For this review, take the finished solid that the model builds, in its own axes (mm). A direction names the side the tool comes from. Coordinates: 2 decimals unless noted, no trailing zeros. Write each loop counter-clockwise with the first axis right and the second up, starting at its lowest first coordinate (ties: lowest second). Pieces come first, ordered by that corner, then holes. Notation, with made-up numbers: (-32, 76.25) -> (2, 76.25) arc R18 ccw to (2, 93.25) -> close; hole circle Ø4 at (-1, -20). An arc over 180 degrees is marked (long way). One line per item, written item: value. Start each with the question number.
1) Add section A-A (x = 300.75). State how many separate pieces and enclosed holes the cut face has, and give its area (3 significant figures).
2) Add section D-D (x = 36). State the section outline as (y, z) points.
3) Mouldability with a two-part tool opening along Y and no side actions: class faces 6 (the flat face through (149, 220, 20)), 7 (the flat face through (115, 0.25, 2)), 8 (the flat face through (209, -4, 40)) as released by +Y, released by -Y, zero draft, split by the parting line, or undercut.
4) For pin 1 Ø6 at (x, z) = (243, 10.5) entering from -Y; pin 2 Ø5 at (x, z) = (136.66, 36.28) entering from +Y; pin 3 Ø6 at (x, y) = (144, 62) entering from +Z; pin 4 Ø10 at (x, z) = (360, 27.5) entering from +Y, all flat-tipped, find the tip position at first contact; note any pin that passes through.
5) Machinability: for faces 1 (the flat face through (424.5, 108, 20)), 2 (the flat face through (213, -5, 41)), 3 (the flat face through (215, 225, 1)), 4 (the flat face through (420, -4, 0.75)), 5 (the flat face through (424.75, 109, 20)), which of the approach directions +Z, -Z, +X, -X, +Y, -Y give a long, thin tool a straight path to every point of the face, cutting with its end or side? Answer none if there is none.
6) For probe 1 along Y at (x, z) = (92, 36); probe 2 along X at (y, z) = (16.5, 38.5); probe 3 along Y at (x, z) = (68.5, 21.5), list the stretches that pass through material, from the lowest coordinate up. Write a range as from..to.
7) Add section C-C (y = 106.5). State the section outline as (x, z) points.
from build123d import *

# Parameters (mm, degrees)
F0_W      = 425
F0_H      = 220
F0_W_2    = 424.5
F0_H_2    = 219.5
F1_DEPTH  = 0.25
F2_DEPTH  = 41
F3_R      = 19
F3_W      = 76
F3_H      = 36
F3_R_2    = 2
F5_DEPTH  = 1
F4_W      = 158
F4_H      = 38.25
F4_W_2    = 120
F4_H_2    = 15
F6_DEPTH  = 1
F8_DEPTH  = 9
F9_R      = 2.75
F9_R_2    = 1.5
F10_DEPTH = 5
F11_W     = 424.75
F11_H     = 41
F11_W_2   = 422.750026226
F11_H_2   = 39.000026226
F12_DEPTH = 10
F13_R     = 2
F14_DEPTH = 0.25


with BuildPart() as f1:
    # F0 (on Top) → F1 (new body)
    with BuildSketch(Plane.XY):
        with Locations((212.25, 110)):
            Rectangle(F0_W, F0_H)
        with Locations((212.25, 110)):
            Rectangle(F0_W_2, F0_H_2, mode=Mode.SUBTRACT)
        with Locations((212.25, 110)):
            Rectangle(F0_W_2, F0_H_2)
    extrude(amount=-F1_DEPTH)

    # F0 (on Top) → F2 (join)
    with BuildSketch(Plane.XY):
        with Locations((212.25, 110)):
            Rectangle(F0_W, F0_H)
        with Locations((212.25, 110)):
            Rectangle(F0_W_2, F0_H_2, mode=Mode.SUBTRACT)
    extrude(amount=F2_DEPTH)

    # F3 (on face) → F5 (cut)
    with BuildSketch(Plane.XZ):
        with Locations((120.75, 20.375)):
            Circle(F3_R)
        with Locations((255.75, 20.375)):
            Circle(F3_R)
        with Locations((300.75, 20.375)):
            Circle(F3_R)
        with Locations((377.75, 19)):
            Rectangle(F3_W, F3_H)
        with Locations((104.8400974233, 36.2849025767)):
            Circle(F3_R_2)
        with Locations((104.8400974233, 4.4650974233)):
            Circle(F3_R_2)
        with Locations((271.6599025767, 36.2849025767)):
            Circle(F3_R_2)
        with Locations((271.6599025767, 4.4650974233)):
            Circle(F3_R_2)
        with Locations((136.6599025767, 36.2849025767)):
            Circle(F3_R_2)
        with Locations((136.6599025767, 4.4650974233)):
            Circle(F3_R_2)
        with Locations((239.8400974233, 36.2849025767)):
            Circle(F3_R_2)
        with Locations((239.8400974233, 4.4650974233)):
            Circle(F3_R_2)
        with Locations((284.8400974233, 36.2849025767)):
            Circle(F3_R_2)
        with Locations((284.8400974233, 4.4650974233)):
            Circle(F3_R_2)
        with Locations((316.6599025767, 36.2849025767)):
            Circle(F3_R_2)
        with Locations((316.6599025767, 4.4650974233)):
            Circle(F3_R_2)
    extrude(amount=-F5_DEPTH, mode=Mode.SUBTRACT)

    # F4 (on face) → F6 (cut)
    with BuildSketch(Plane(origin=(0, 220, 0), x_dir=(-1, 0, 0), z_dir=(0, 1, 0))):
        Polygon((-384.75, 34.75), (-414.75, 34.75), (-414.75, 1.75), (-338.75, 1.75), (-338.75, 30), (-342.75, 30), (-342.75, 40), (-384.75, 40), align=None)
        with Locations((-243.25, 20.875)):
            Rectangle(F4_W, F4_H)
        with Locations((-74.25, 22.5)):
            Rectangle(F4_W_2, F4_H_2)
    extrude(amount=-F6_DEPTH, mode=Mode.SUBTRACT)

    # F7 (on face) → F8 (join)
    with BuildSketch(Plane.XZ):
        Polygon((424.75, 41), (-0.25, 41), (-0.25, -0.25), (339.75, -0.25), (339.75, 0.7500000065), (0.7500000065, 0.7500000065), (0.7500000065, 39.9999999935), (423.7499999935, 39.9999999935), (423.7499999935, 0.7500000065), (415.75, 0.7500000065), (415.75, -0.25), (424.75, -0.25), align=None)
    extrude(amount=F8_DEPTH)

    # F9 (on face) → F10 (join)
    with BuildSketch(Plane.XY):
        with Locations((156.25, 207.75)):
            Circle(F9_R)
        with Locations((156.25, 207.75)):
            Circle(F9_R_2, mode=Mode.SUBTRACT)
        with Locations((313.73, 184.89)):
            Circle(F9_R)
        with Locations((313.73, 184.89)):
            Circle(F9_R_2, mode=Mode.SUBTRACT)
        with Locations((156.25, 52.81)):
            Circle(F9_R)
        with Locations((156.25, 52.81)):
            Circle(F9_R_2, mode=Mode.SUBTRACT)
        with Locations((313.73, 52.81)):
            Circle(F9_R)
        with Locations((313.73, 52.81)):
            Circle(F9_R_2, mode=Mode.SUBTRACT)
    extrude(amount=F10_DEPTH)

    # F11 (on face) → F12 (join)
    with BuildSketch(Plane(origin=(0, 220, 0), x_dir=(-1, 0, 0), z_dir=(0, 1, 0))):
        with Locations((-212.375, 20.5)):
            Rectangle(F11_W, F11_H)
        with Locations((-212.375, 20.5)):
            Rectangle(F11_W_2, F11_H_2, mode=Mode.SUBTRACT)
    extrude(amount=F12_DEPTH)

    # F13 (on face) → F14 (cut, through all)
    with BuildSketch(Plane.XY):
        with Locations((340.75, 63.25)):
            Circle(F13_R)
        with Locations((411.75, 63.25)):
            Circle(F13_R)
    extrude(amount=-F14_DEPTH, mode=Mode.SUBTRACT)


solid = f1.part
Numbers:
1. separate pieces: 3
1. enclosed holes: 0
1. area: 94.4 mm²
2. outline: (-9, -0.25) -> (220, -0.25) -> (220, 0) -> (230, 0) -> (230, 1) -> (220, 1) -> (220, 15) -> (219.75, 15) -> (219.75, 0) -> (0.25, 0) -> (0.25, 41) -> (-9, 41) -> (-9, 40) -> (0, 40) -> (0, 0.75) -> (-9, 0.75) -> close; (219.75, 30) -> (220, 30) -> (220, 40) -> (230, 40) -> (230, 41) -> (219.75, 41) -> close
3. face 6: released by +Y
3. face 7: undercut
3. face 8: zero draft
4. pin 1: y = 0
4. pin 2: y = 220
4. pin 3: z = 0
4. pin 4: through
5. face 1: +Z
5. face 2: +Z, +X, -X, +Y, -Y
5. face 3: +Y
5. face 4: -Y
5. face 5: +Z, -Z, +X, +Y, -Y
6. probe 1: 0..0.25, 219.75..220
6. probe 2: -0.25..0, 424.5..424.75
6. probe 3: 0..0.25
7. outline: (-0.25, -0.25) -> (424.75, -0.25) -> (424.75, 41) -> (424.5, 41) -> (424.5, 0) -> (0, 0) -> (0, 41) -> (-0.25, 41) -> close
